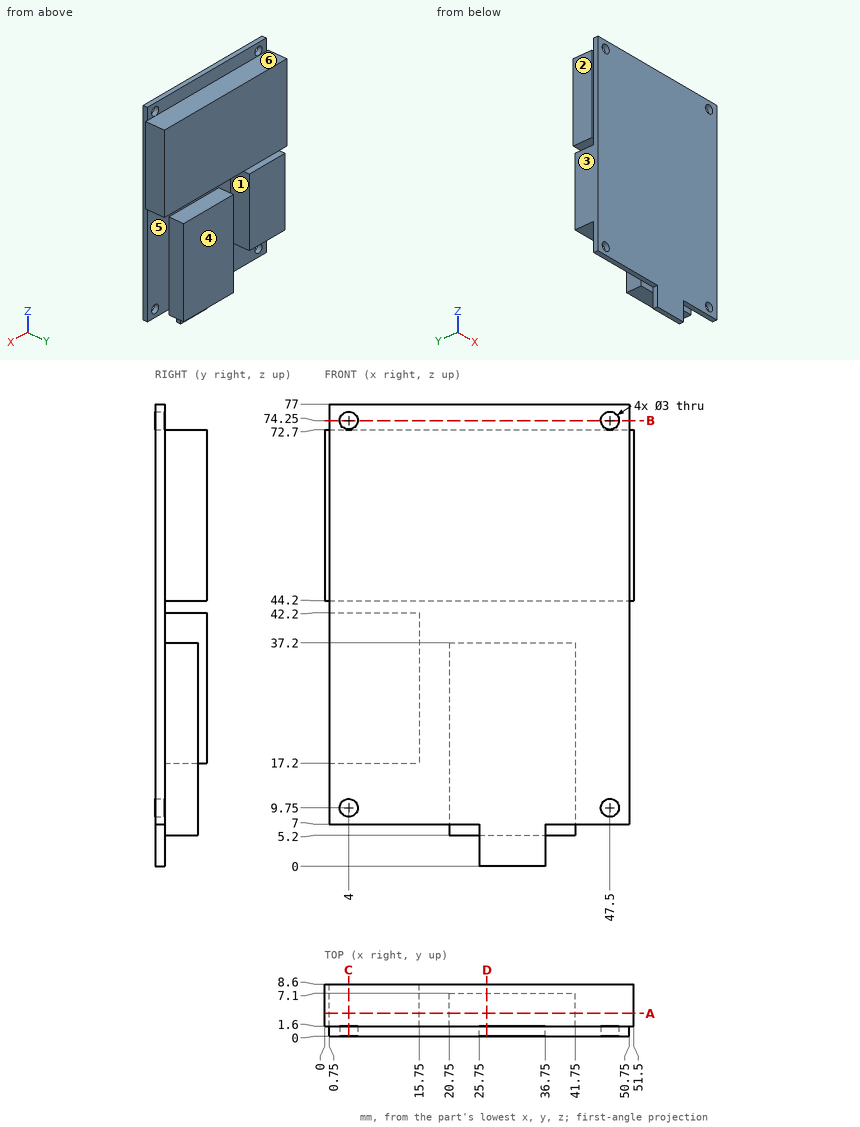
Could you check a few things on this drawing? It's one solid part, dimensions in mm from its lowest x, y, z. A direction names the side the tool comes from. Give positions to 0.01 mm unless a question says otherwise; leave off trailing zeros. Order: outer loops, then holes, each group sorted by start corner. A loop starts at its lowest first (then second) coordinate and runs counter-clockwise, first axis right, second up. Notation, with made-up numbers: (-28, -20.75) - (-11, -20.75) arc R14 cw to (-11, -0.75) - close; hole circle Ø10 at (64, 42). An arc over 180 degrees is marked (long way). Return JSON: item names as keys, results as strings. Group by question number.
Q1. Suppose I cut it at B-B, the plane z = 74.25. Please give me the cut outline in (x, y).
Q2. Will these pins go through, and if not, where does the flat tip stop? pin 1 Ø4.5 at (x, y) = (32.5, 5.5) entering from +Z; pin 2 Ø3 at (y, z) = (5, 32.5) entering from +X; pin 3 Ø2 at (x, y) = (14.5, 4) entering from -Z.
Q3. Suppose I cut it at C-C, the plane x = 4. Please give me the cut outline in (y, z).
Q4. Please list where these lines run through material, in increasing order: line 1 along Z through (x, y) = (47.5, 0.5); line 2 along X through (y, z) = (1.2, 9.75); line 3 along Z through (x, y) = (38, 2.25). Write a range as [from, to].
Q5. Thinking about a two-plate mould opening in Z: for the marked faces 4, 5 and 6, which applies, pulls with the +Z half, pulls with the -Z half, needs draft (parallel to the pull), parting line crosses it, or undercut?
Q6. Suppose I cut it at D-D, the plane x = 27. Please give me the cut outline in (y, z).
Q7. Suppose I cut it at A-A, the plane y = 3.75. Please give me the cut outline in (x, z).
Q8. Which directions (+Z, -Z, +X, -X, +Y, -Y) give clear straight access to the entire face, cutting with the end or side of a thin tool? Please do the marked faces 1, 2 and 3.
Resolved:
{
 "1": {"outline": "(0.75, 0) - (2.5, 0) - (2.5, 1.6) - (0.75, 1.6) - close; (5.5, 0) - (46, 0) - (46, 1.6) - (5.5, 1.6) - close; (49, 0) - (50.75, 0) - (50.75, 1.6) - (49, 1.6) - close"},
 "2": {"pin 1": "stops at z = 72.7", "pin 2": "stops at x = 41.75", "pin 3": "stops at z = 17.2"},
 "3": {"outline": "(0, 7) - (1.6, 7) - (1.6, 8.25) - (0, 8.25) - close; (0, 11.25) - (1.6, 11.25) - (1.6, 17.2) - (8.6, 17.2) - (8.6, 42.2) - (1.6, 42.2) - (1.6, 44.2) - (8.6, 44.2) - (8.6, 72.7) - (1.6, 72.7) - (1.6, 72.75) - (0, 72.75) - close; (0, 75.75) - (1.6, 75.75) - (1.6, 77) - (0, 77) - close"},
 "4": {"line 1": "z = [7, 8.25], [11.25, 72.75], [75.75, 77]", "line 2": "x = [0.75, 2.5], [5.5, 46], [49, 50.75]", "line 3": "z = [5.2, 37.2], [44.2, 72.7]"},
 "5": {"face 4": "needs draft", "face 5": "undercut", "face 6": "pulls with the +Z half"},
 "6": {"outline": "(0, 0) - (1.6, 0) - (1.6, 5.2) - (7.1, 5.2) - (7.1, 37.2) - (1.6, 37.2) - (1.6, 44.2) - (8.6, 44.2) - (8.6, 72.7) - (1.6, 72.7) - (1.6, 77) - (0, 77) - close"},
 "7": {"outline": "(0, 44.2) - (51.5, 44.2) - (51.5, 72.7) - (0, 72.7) - close; (0.75, 17.2) - (15.75, 17.2) - (15.75, 42.2) - (0.75, 42.2) - close; (20.75, 5.2) - (41.75, 5.2) - (41.75, 37.2) - (20.75, 37.2) - close"},
 "8": {"face 1": "-Z, +Y", "face 2": "+Z, -Z, -X, +Y, -Y", "face 3": "-Z, -X, -Y"}
}
